from build123d import *

# Parameters (mm, degrees)
BOSS_EXTRUDE1_DEPTH = 800
SKETCH3_R           = 30
BOSS_EXTRUDE3_DEPTH = 20
SKETCH4_R           = 30
CUT_EXTRUDE1_DEPTH  = 1391.647331281
SKETCH5_R           = 15
BOSS_EXTRUDE4_DEPTH = 100
SKETCH6_R           = 30
CUT_EXTRUDE2_DEPTH  = 20
BOSS_EXTRUDE5_START = -140
SKETCH7_R           = 30
BOSS_EXTRUDE5_DEPTH = 20


with BuildPart() as part:
    # Sketch1 → Boss-Extrude1 (new, symmetric)
    with BuildSketch(Plane.XY):
        with BuildLine():
            Line((-5, 14.142135624), (-5, 18.3))
            Line((-5, 18.3), (5, 18.3))
            Line((5, 18.3), (5, 14.142135624))
            ThreePointArc((5, 14.142135624), (0, -15), (-5, 14.142135624))
        make_face()
    extrude(amount=BOSS_EXTRUDE1_DEPTH, both=True)

    # Sketch3 → Boss-Extrude3 (add)
    with BuildSketch(Plane(origin=(0, 0, 590), x_dir=(-1, 0, 0), z_dir=(0, 0, -1))):
        Circle(SKETCH3_R)
    boss_extrude3 = extrude(amount=-BOSS_EXTRUDE3_DEPTH)

    # Mirror2: Boss-Extrude3 across plane
    add(boss_extrude3.mirror(Plane.XY))

    # Sketch4 → Cut-Extrude1 (cut, through all)
    with BuildSketch(Plane.XY.offset(-590)):
        with Locations(Location((0, 0, 0), (0, 0, 180))):
            Circle(SKETCH4_R)
    extrude(amount=CUT_EXTRUDE1_DEPTH, mode=Mode.SUBTRACT)

    # Sketch5 → Boss-Extrude4 (add)
    with BuildSketch(Plane(origin=(0, 0, -800), x_dir=(-1, 0, 0), z_dir=(0, 0, -1))):
        Circle(SKETCH5_R)
    extrude(amount=BOSS_EXTRUDE4_DEPTH)

    # Sketch6 → Cut-Extrude2 (cut)
    with BuildSketch(Plane.XY.offset(-590)):
        Circle(SKETCH6_R)
    extrude(amount=-CUT_EXTRUDE2_DEPTH, mode=Mode.SUBTRACT)

    # Sketch7 → Boss-Extrude5 (add)
    with BuildSketch(Plane.XY.offset(-610).offset(BOSS_EXTRUDE5_START)):
        Circle(SKETCH7_R)
    extrude(amount=BOSS_EXTRUDE5_DEPTH)


solid = part.part
Work out the finished part from the listing and answer in its coordinate system (mm). A direction names the side the tool comes from. Round coordinates to 2 decimals unless told otherwise and drop trailing zeros. Loops run counter-clockwise (first coordinate to the right, second up) from the corner with the lowest first, then second, coordinate; pieces in that order, holes last. Notation, with made-up numbers: (28, 86) - (51, 86) arc R12 cw to (51, 103) - close; hole circle Ø5 at (79, 7.5). An arc over 180 degrees is marked (long way). Use one line per item in the form item = value. Start each with the question number.
(1) Consider line 1 (Z direction, x = -4.5, y = -17.5); line 2 (Y direction, x = 1, z = -777.5); line 3 (X direction, y = -11.5, z = -707). Determine where each line is inside the solid, lowest interval first.
(2) Find section C-C on z = -860.5. Determine the outline of the cut face in (x, y).
(3) Flat-ended cylindrical pins translate along their axes: P1, Ø1.5, axis at y = -9.5, z = -676.5, coming from the -X side; P2, Ø4.5, axis at y = 16, z = -767, coming from the +X side; P3, Ø11, axis at x = 1, z = -677, coming from the +Y side. Find the tip coordinate at first contact, or state that the pin passes through.
(4) Which of the six approach directions +Z, -Z, +X, -X, +Y, -Y give full straight-line access (tool end or side, diameter ignored) to faces 1 (the face through (0, 18.3, -775)), 2 (the face through (0, 18.3, -669)), 3 (the face through (0.59, -14.99, -669.16))?
(5) Find section A-A on y = 0. Determine the outline of the cut face in (x, z), and give its area (3 significant figures).
(6) Find section B-B on x = 0. Determine the outline of the cut face in (y, z).
(7) Find section D-D on z = -704.5. Determine the outline of the cut face in (x, y).
Answer list:
q1.line_1 = -750 to -730
q1.line_2 = -14.97 to 18.3
q1.line_3 = -9.63 to 9.63
q2.outline = circle Ø30 at (0, 0)
q3.P1 = -12.18
q3.P2 = 5.99
q3.P3 = 18.3
q4.face_1 = -Z, +X, -X, +Y
q4.face_2 = +Z, +X, -X, +Y
q4.face_3 = +Z
q5.outline = (-30, -750) - (-15, -750) - (-15, -900) - (15, -900) - (15, -750) - (30, -750) - (30, -730) - (15, -730) - (15, -610) - (-15, -610) - (-15, -730) - (-30, -730) - close
q5.area = 9,300 mm^2
q6.outline = (-30, -750) - (-15, -750) - (-15, -900) - (15, -900) - (15, -800) - (18.3, -800) - (18.3, -750) - (30, -750) - (30, -730) - (18.3, -730) - (18.3, -610) - (-15, -610) - (-15, -730) - (-30, -730) - close
q7.outline = (-5, 14.14) arc R15 ccw (long way) to (5, 14.14) - (5, 18.3) - (-5, 18.3) - close
